```python
from build123d import *

# Parameters (mm, degrees)
SKETCH1_W                      = 50.8
SKETCH1_H                      = 19.05
BOSS_EXTRUDE1_DEPTH            = 9.525
F_1_2_0_5_DIAMETER_HOLE1_D     = 12.7
F_1_2_0_5_DIAMETER_HOLE1_DEPTH = 70.104
F_1_2_0_5_DIAMETER_HOLE1_TIP   = 3.815464931
F_10_32_TAPPED_HOLE1_D         = 4.0386
F_10_32_TAPPED_HOLE1_DEPTH     = 11.938
F_10_32_TAPPED_HOLE1_TIP       = 1.213317848


with BuildPart() as part:
    # Sketch1 → Boss-Extrude1 (new body)
    with BuildSketch(Plane(origin=(0, 0, 0), x_dir=(0, 0, -1), z_dir=(1, 0, 0))):
        Rectangle(SKETCH1_W, SKETCH1_H)
    extrude(amount=BOSS_EXTRUDE1_DEPTH)

    # 1/2 (0.5) Diameter Hole1
    with Locations(Plane(origin=(9.525, 0, 0), x_dir=(0, 0, -1), z_dir=(1, 0, 0))):
        with Locations((0, 1.905)):
            Hole(F_1_2_0_5_DIAMETER_HOLE1_D / 2, depth=F_1_2_0_5_DIAMETER_HOLE1_DEPTH)
            with Locations((0, 0, -(F_1_2_0_5_DIAMETER_HOLE1_DEPTH + F_1_2_0_5_DIAMETER_HOLE1_TIP / 2))):  # 118° drill point
                Cone(0, F_1_2_0_5_DIAMETER_HOLE1_D / 2, F_1_2_0_5_DIAMETER_HOLE1_TIP, mode=Mode.SUBTRACT)

    # #10-32 Tapped Hole1
    with Locations(Plane(origin=(-1.022565875, -1.088669914, -25.4), x_dir=(-1, 0, 0), z_dir=(0, 0, -1))):
        with Locations((-5.785065875, -2.086330086), (-5.785065875, 6.803669914)):
            Hole(F_10_32_TAPPED_HOLE1_D / 2, depth=F_10_32_TAPPED_HOLE1_DEPTH)
            with Locations((0, 0, -(F_10_32_TAPPED_HOLE1_DEPTH + F_10_32_TAPPED_HOLE1_TIP / 2))):  # 118° drill point
                Cone(0, F_10_32_TAPPED_HOLE1_D / 2, F_10_32_TAPPED_HOLE1_TIP, mode=Mode.SUBTRACT)


solid = part.part
```
Input: part model. Units: mm. Frame: model coordinates. A direction names the side the tool comes from. Give positions to 0.01 mm unless a question says otherwise; leave off trailing zeros. Write each loop counter-clockwise with the first axis right and the second up, starting at its lowest first coordinate (ties: lowest second). Pieces come first, ordered by that corner, then holes. Notation, with made-up numbers: (9, 9.5) - (15, 9.5) arc R26 cw to (15, 34.5) - close; hole circle Ø2 at (31.5, 70.25). An arc over 180 degrees is marked (long way). Write item = value, one per line. Start each with the question number.
1) Cut plane D-D (x = 8). Return loops of the section in (y, z) (3 decimals).
2) Draft query along Z for faces 1 (the face through (4.696, 3.812, 6.057)), 2 (the face through (5, 0, 25.4)), 3 (the face through (5, 0, -25.4)), 4 (the face through (0, -2, 6)). Return one class per face: pulls with the +Z half, pulls with the -Z half, needs draft (parallel to the pull), parting line crosses it, or undercut.
3) Cut plane C-C (z = -17). Return loops of the section in (x, y) (1 decimal), and give its area (3 significant figures).
4) Reachability of faces 5 (the face through (3.274, 7.08, -19.347)), 6 (the face through (5, -9.525, 0)) from +Z, -Z, +X, -X, +Y, -Y: full face, straight path, thin tool, end or side. Return the list, or none.
5) Material intervals for L1, parallel to Y at x = 5, z = 0 (3 decimals); L2, parallel to Z at x = 2.5, y = 2; L3, parallel to Y at x = 5.5, z = -20 (3 decimals), sorted ascending. Write a range as [from, to].
6) Cut plane B-B (y = 0.75). Return loops of the section in (x, z) (3 decimals), and give its area (3 significant figures).
7) Cut plane A-A (z = -1). Return loops of the section in (x, y) (3 decimals), and give its area (3 significant figures).
Answers follow:
q1.outline = (-9.525, -25.4) - (9.525, -25.4) - (9.525, 25.4) - (-9.525, 25.4) - close; hole circle Ø12.7 at (1.905, 0)
q2.face_1 = undercut
q2.face_2 = pulls with the +Z half
q2.face_3 = pulls with the -Z half
q2.face_4 = needs draft
q3.outline = (0, -9.5) - (9.5, -9.5) - (9.5, 9.5) - (0, 9.5) - close; hole circle Ø4 at (4.8, -3.2); hole circle Ø4 at (4.8, 5.7)
q3.area = 156 mm^2
q4.face_5 = -Z
q4.face_6 = +Z, -Z, +X, -X, -Y
q5.L1 = [-9.525, -4.445], [8.255, 9.525]
q5.L2 = [-25.4, -6.35], [6.35, 25.4]
q5.L3 = [-9.525, -5.055], [-1.295, 3.835], [7.595, 9.525]
q6.outline = (0, -25.4) - (9.525, -25.4) - (9.525, -6.244) - (0, -6.244) - close; (0, 6.244) - (9.525, 6.244) - (9.525, 25.4) - (0, 25.4) - close
q6.area = 365 mm^2
q7.outline = (0, -9.525) - (9.525, -9.525) - (9.525, -4.366) - (0, -4.366) - close; (0, 8.176) - (9.525, 8.176) - (9.525, 9.525) - (0, 9.525) - close
q7.area = 62.0 mm^2
